from build123d import *

# Parameters (mm, degrees)
F1_DEPTH  = 100
F2_R      = 3
F3_DEPTH  = 105.001
F4_W      = 66
F4_H      = 70
F5_DEPTH  = 25
F6_W      = 3
F6_H      = 15
F7_DEPTH  = 29
F8_W      = 15
F8_H      = 3
F9_DEPTH  = 3
F10_W     = 15
F10_H     = 3
F11_DEPTH = 3
F12_R     = 1
F13_R     = 2
F14_R     = 5


with BuildPart() as f1:
    # F0 (on Front) → F1 (new body)
    with BuildSketch(Plane.XZ):
        Polygon((105, 27), (0, 27), (0, 0), (3, 0), (3, 24), (102, 24), (102, 0), (105, 0), align=None)
    extrude(amount=F1_DEPTH)

    # F2 (on face) → F3 (cut, through all)
    with BuildSketch(Plane.YZ.offset(105)):
        with Locations((-7, 5)):
            Circle(F2_R)
        with Locations((-49, 5)):
            Circle(F2_R)
    extrude(amount=-F3_DEPTH, mode=Mode.SUBTRACT)

    # F4 (on face) → F5 (cut)
    with BuildSketch(Plane.XY.offset(27)):
        with Locations((52.5, -35)):
            Rectangle(F4_W, F4_H)
    extrude(amount=-F5_DEPTH, mode=Mode.SUBTRACT)

    # F6 (on face) → F7 (join)
    with BuildSketch(Plane.XY.offset(27)):
        with Locations((18, -7.5)):
            Rectangle(F6_W, F6_H)
        with Locations((18, -52.5)):
            Rectangle(F6_W, F6_H)
        with Locations((87, -7.5)):
            Rectangle(F6_W, F6_H)
        with Locations((87, -52.5)):
            Rectangle(F6_W, F6_H)
    extrude(amount=F7_DEPTH)

    # F8 (on face) → F9 (join)
    with BuildSketch(Plane.YZ.offset(19.5)):
        with Locations((-52.5, 54.5)):
            Rectangle(F8_W, F8_H)
        with Locations((-7.5, 54.5)):
            Rectangle(F8_W, F8_H)
    extrude(amount=F9_DEPTH)

    # F10 (on face) → F11 (join)
    with BuildSketch(Plane(origin=(85.5, 0, 0), x_dir=(0, -1, 0), z_dir=(-1, 0, 0))):
        with Locations((7.5, 54.5)):
            Rectangle(F10_W, F10_H)
        with Locations((52.5, 54.5)):
            Rectangle(F10_W, F10_H)
    extrude(amount=F11_DEPTH)

    # F12
    f12_edges = [f1.edges().sort_by_distance(p)[0] for p in [
        (3, -50, 24),
        (102, -50, 24),
        (16.5, -7.5, 27),
        (18, -15, 27),
        (16.5, -52.5, 27),
        (18, -60, 27),
        (18, -45, 27),
        (87, -60, 27),
        (88.5, -52.5, 27),
        (87, -15, 27),
        (88.5, -7.5, 27),
        (87, -45, 27),
    ]]
    fillet(f12_edges, radius=F12_R)

    # F13
    f13_edges = [f1.edges().sort_by_distance(p)[0] for p in [
        (0, -50, 27),
        (105, -50, 27),
    ]]
    fillet(f13_edges, radius=F13_R)

    # F14
    f14_edges = [f1.edges().sort_by_distance(p)[0] for p in [
        (85.5, -70, 25.5),
        (19.5, -70, 25.5),
    ]]
    fillet(f14_edges, radius=F14_R)


solid = f1.part
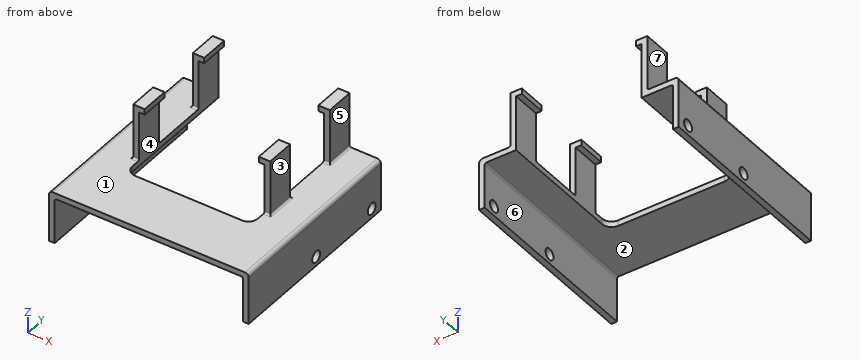
Read the model definition and answer for the solid it produces. Units are mm, in the model's axes. Face numbers are marked on the shaded views. A direction names the side the tool comes from. Give positions to 0.01 mm unless a question says otherwise; leave off trailing zeros. Write each loop counter-clockwise with the first axis right and the second up, starting at its lowest first coordinate (ties: lowest second). Pieces come first, ordered by that corner, then holes. Notation, with made-up numbers: (69, -21.75) - (93, -21.75) arc R11 ccw to (93, -4.75) - close; hole circle Ø7 at (71.5, 78.25). An arc over 180 degrees is marked (long way). Use CSV: the item, a comma, the result in double quotes. Start each with the question number.
Item 1: The part is cut by section C-C, the plane z = 40. Give the vertices of the cut face in (x, y).
Item 2: The part is cut by section D-D, the plane y = -33. Give the vertices of the cut face in (x, z).
Item 3: Flat-ended cylindrical pins translate along their axes: P1, Ø16.5, axis at y = -4.5, z = 39, coming from the +X side; P2, Ø8, axis at x = 20, y = -24.5, coming from the +Z side; P3, Ø0.9, axis at x = 20.5, y = -10.5, coming from the -Z side. Find the tip coordinate at first contact, or state that the pin passes through.
Item 4: The part is cut by section B-B, the plane y = -49. Count the separate pieces of the cut face and the enclosed holes in it, and give its area (3 significant figures).
Item 5: The part is cut by section A-A, the plane z = 21.5. Give the vertices of the cut face in (x, y), and give its area (3 significant figures).
Item 6: The mould has two halves that part along X. Classify the marked faces 1, 2 and 3: pulls with the +X half, pulls with the -X half, needs draft (parallel to the pull), parting line crosses it, or undercut.
Item 7: For the marked faces 4, 5, 6 and 7, determine the directions among +Z, -Z, +X, -X, +Y, -Y from which every point of the face is accessible in a straight line to the end or side of a thin tool.
Item 8: Consider line 1 (X direction, y = -52, z = 30.5); line 2 (X direction, y = -93.5, z = 6); line 3 (Z direction, x = 2.35, y = -49). Determine where each line is inside the solid, lowest interval first.
Taken from the geometry:
1,outline,"(16.5, -60) - (19.5, -60) - (19.5, -45) - (16.5, -45) - close; (16.5, -15) - (19.5, -15) - (19.5, 0) - (16.5, 0) - close; (85.5, -60) - (88.5, -60) - (88.5, -45) - (85.5, -45) - close; (85.5, -15) - (88.5, -15) - (88.5, 0) - (85.5, 0) - close"
2,outline,"(0, 0) - (3, 0) - (3, 23) arc R1 cw to (4, 24) - (19.5, 24) - (19.5, 27) - (2, 27) arc R2 ccw to (0, 25) - close; (85.5, 24) - (101, 24) arc R1 cw to (102, 23) - (102, 0) - (105, 0) - (105, 25) arc R2 ccw to (103, 27) - (85.5, 27) - close"
3,P1,"x = 88.5"
3,P2,"z = 27"
3,P3,"z = 53"
4,separate pieces,"4"
4,enclosed holes,"0"
4,area,"416 mm2"
5,outline,"(0, -100) - (3, -100) - (3, 0) - (0, 0) - close; (102, -100) - (105, -100) - (105, 0) - (102, 0) - close"
5,area,"600 mm2"
6,face 1,"needs draft"
6,face 2,"undercut"
6,face 3,"pulls with the +X half"
7,face 4,"-Z, +Y"
7,face 5,"+Z, +X, +Y, -Y"
7,face 6,"-Z, +Y, -Y"
7,face 7,"+Z, -X, +Y, -Y"
8,line 1,"16.5 to 19.5, 85.5 to 88.5"
8,line 2,"0 to 3, 102 to 105"
8,line 3,"0 to 2, 8 to 27"
